Source: three-view drawing plus pictorial views. Frame: mm from the lowest corner of the part. Coordinates: 2 decimals unless noted, no trailing zeros. Loops run counter-clockwise (first coordinate to the right, second up) from the corner with the lowest first, then second, coordinate; pieces in that order, holes last. Notation, with made-up numbers: (51, -27.5) - (58, -27.5) arc R15 cw to (58, -14.5) - close; hole circle Ø11 at (35, 49). An arc over 180 degrees is marked (long way). Use CSV: the item, a comma, the result in double quotes. Start each with the question number.
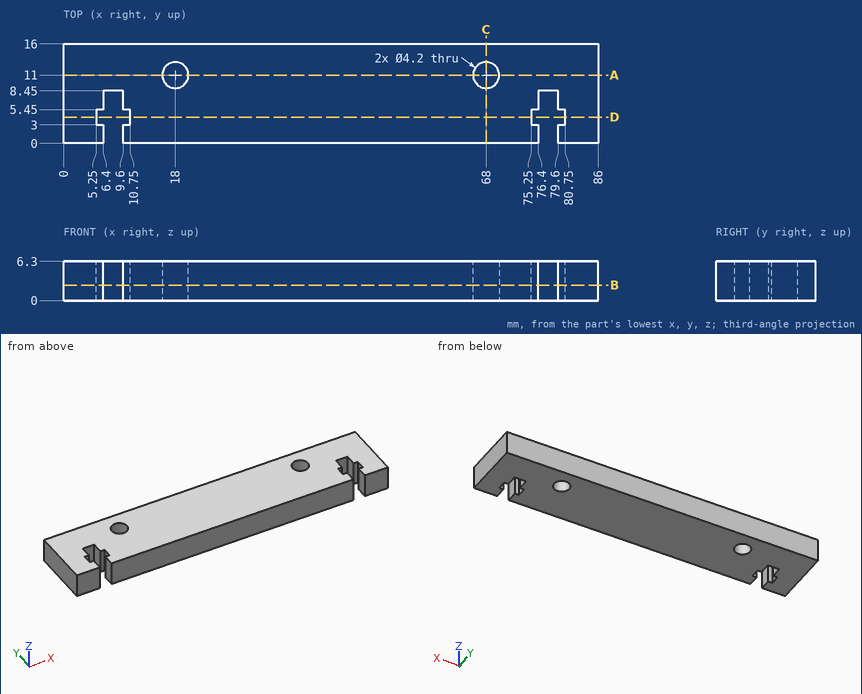
(1) Section C-C on x = 68. Output: boundary loops of the cut face in (y, z), plus the area to 3 significant figures.
(2) Ray query, line 1 (X direction, y = 2, z = 0.5); line 2 (Y direction, x = 68, z = 2); line 3 (Y direction, x = 10.5, z = 1.5). Return the intervals inside material, ascending. Write a range as [from, to].
(3) Section A-A on y = 11. Output: boundary loops of the cut face in (x, z), plus the area to 3 significant figures.
(4) Section B-B on z = 2.5. State how many separate pieces and enclosed holes the cut face has, plus the area to 3 significant figures.
(5) Pin query (flat end, axial travel): pin 1 Ø0.6 at (x, z) = (6, 2.5) entering from -Y. Return the tip coordinate at first contact, or that it passes through.
(6) Section D-D on y = 4.25. Output: boundary loops of the cut face in (x, z).
Solution:
1,outline,"(0, 0) - (8.9, 0) - (8.9, 6.3) - (0, 6.3) - close; (13.1, 0) - (16, 0) - (16, 6.3) - (13.1, 6.3) - close"
1,area,"74.3 mm²"
2,line 1,"x = [0, 6.4], [9.6, 76.4], [79.6, 86]"
2,line 2,"y = [0, 8.9], [13.1, 16]"
2,line 3,"y = [0, 3], [5.45, 16]"
3,outline,"(0, 0) - (15.9, 0) - (15.9, 6.3) - (0, 6.3) - close; (20.1, 0) - (65.9, 0) - (65.9, 6.3) - (20.1, 6.3) - close; (70.1, 0) - (86, 0) - (86, 6.3) - (70.1, 6.3) - close"
3,area,"489 mm²"
4,separate pieces,"1"
4,enclosed holes,"2"
4,area,"1,280 mm²"
5,pin 1,"stops at y = 0"
6,outline,"(0, 0) - (5.25, 0) - (5.25, 6.3) - (0, 6.3) - close; (10.75, 0) - (75.25, 0) - (75.25, 6.3) - (10.75, 6.3) - close; (80.75, 0) - (86, 0) - (86, 6.3) - (80.75, 6.3) - close"
